CAD build for the part. Positions are in the model's coordinates, mm. Face numbers are marked on the shaded views. A direction names the side the tool comes from. Give positions to 0.01 mm unless a question says otherwise; leave off trailing zeros. Loops run counter-clockwise (first coordinate to the right, second up) from the corner with the lowest first, then second, coordinate; pieces in that order, holes last. Notation, with made-up numbers: M 15.25,39.25 L 46.25,39.25 A18 cw 46.25,58.25 Z; hole C 32.25,-4 d4. An arc over 180 degrees is marked long. One line per question, with ' | ' between items.
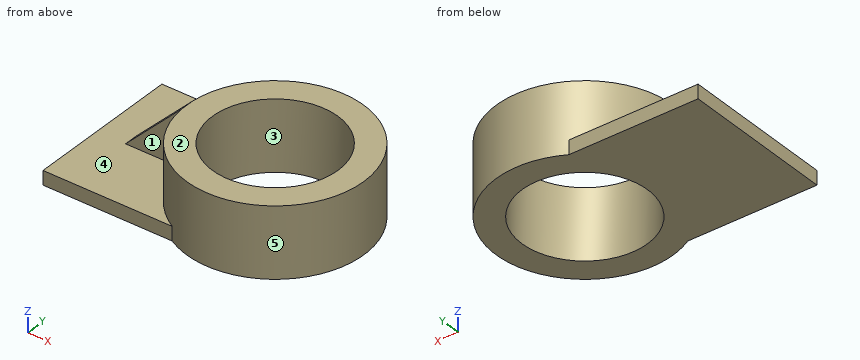
```python
from build123d import *

# Parameters (mm, degrees)
F1_DEPTH = 7.62
F2_R     = 48.082642
F2_R_2   = 34.067148
F3_DEPTH = 38.1
F5_DEPTH = 38.1
F7_DEPTH = 52.059737


with BuildPart() as f1:
    # F0 (on Top) → F1 (new body)
    with BuildSketch(Plane.XY):
        with BuildLine():
            Line((-45.755789, -41.841321), (45.755789, -41.841321))
            ThreePointArc((45.755789, -41.841321), (3.914468, 0), (45.755789, 41.841321))
            Line((45.755789, 41.841321), (-45.755789, 41.841321))
            Line((-45.755789, 41.841321), (-45.755789, -41.841321))
        make_face()
    extrude(amount=F1_DEPTH)

    # F2 (on Top) → F3 (join)
    with BuildSketch(Plane.XY):
        with Locations((48.082642, 0)):
            Circle(F2_R)
        with Locations((48.082642, 0)):
            Circle(F2_R_2, mode=Mode.SUBTRACT)
    extrude(amount=F3_DEPTH)

    # F4 (on face) → F5 (join)
    with BuildSketch(Plane.XY.offset(7.62)):
        with BuildLine():
            Line((0.164679, -3.976095), (0.164679, 3.976095))
            ThreePointArc((0.164679, 3.976095), (0, 0), (0.164679, -3.976095))
        make_face()
        with BuildLine():
            ThreePointArc((0.164679, -3.976095), (0, 0), (0.164679, 3.976095))
            Line((0.164679, 3.976095), (-30.132134, 3.976095))
            Line((-30.132134, 3.976095), (-30.132134, -3.976095))
            Line((-30.132134, -3.976095), (0.164679, -3.976095))
        make_face()
    extrude(amount=F5_DEPTH)

    # F6 (on face) → F7 (cut, through all)
    with BuildSketch(Plane.XZ.offset(3.976095)):
        Polygon((-30.132134, 7.62), (0.164679, 38.1), (0.164679, 45.72), (-30.132134, 45.72), align=None)
    extrude(amount=-F7_DEPTH, mode=Mode.SUBTRACT)


solid = f1.part
```
Item 1: 3-axis set-ups, long thin cutter, end or side, ignore diameter. For the marked faces 1 and 2: which of +Z, -Z, +X, -X, +Y, -Y reach the whole face in a straight line?
Conclusion:
face 1: +Z, -X, -Y | face 2: +Z, +X, -X, +Y, -Y
Item 2: Saw through at D-D on x = -2. Give the cut face in (y, z).
Conclusion:
outline: M -41.84,0 L 41.84,0 L 41.84,7.62 L 3.98,7.62 L 3.98,35.92 L -3.98,35.92 L -3.98,7.62 L -41.84,7.62 Z
Item 3: Drill centre lines: line 1 along Z through (x, y) = (-11.5, 41); line 2 along Y through (x, z) = (44, 17); line 3 along X through (y, z) = (-3, 17). Where is each one in solid material? Low to high. Write a range as [from, to].
Conclusion:
line 1: [0, 7.62] | line 2: [-47.91, -33.82], [33.82, 47.91] | line 3: [-20.81, 14.15], [82.02, 96.07]
Item 4: Saw through at B-B on x = 54.5. Give the cut face in (y, z).
Conclusion:
outline: M -47.65,0 L -33.46,0 L -33.46,38.1 L -47.65,38.1 Z; M 33.46,0 L 47.65,0 L 47.65,38.1 L 33.46,38.1 Z
Item 5: Saw through at A-A on y = 0. Give the cut face in (x, z), and give its area (3 significant figures).
Conclusion:
outline: M -45.76,0 L 14.02,0 L 14.02,38.1 L 0.16,38.1 L -30.13,7.62 L -45.76,7.62 Z; M 82.15,0 L 96.17,0 L 96.17,38.1 L 82.15,38.1 Z | area: 1,870 mm²
Item 6: Mould opens along X. For the marked faces 3, 4 and 5 say: pulls with the +X half, pulls with the -X half, needs draft (parallel to the pull), parting line crosses it, or undercut.
Conclusion:
face 3: undercut | face 4: needs draft | face 5: parting line crosses it
Item 7: Drop flat-ended pins along their axis: P1, Ø8.5, axis at x = -21, z = 4.5, coming from the +Y side; P2, Ø9, axis at x = -17, z = 25.5, coming from the -Y side; P3, Ø4, axis at x = 3.5, y = 21.5, coming from the -Z side; P4, Ø2, axis at x = 40.5, z = 21.5, coming from the -Y side. Give the stop position or say it passes through.
Conclusion:
P1: y = 41.84 | P2: y = -3.98 | P3: z = 0 | P4: y = -47.63
